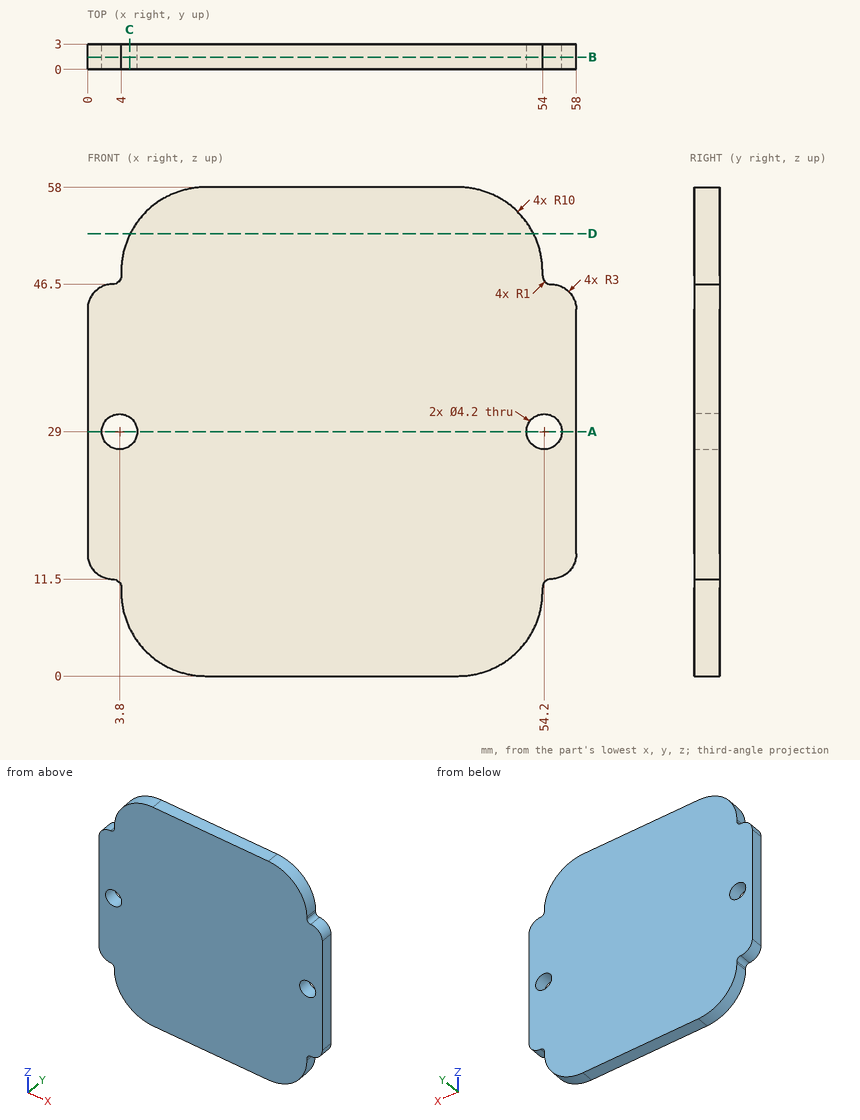
For this review, use the dimensioned drawing (mm, ordinates from the lowest corner) and the shaded views. Coordinates: 2 decimals unless noted, no trailing zeros. Loops run counter-clockwise (first coordinate to the right, second up) from the corner with the lowest first, then second, coordinate; pieces in that order, holes last. Notation, with made-up numbers: (-19.75, 57) - (-8.75, 57) arc R32 ccw to (-8.75, 88) - close; hole circle Ø6 at (26, -0.5). An arc over 180 degrees is marked (long way). Use one line per item in the form item = value. Start each with the question number.
1) Take a section at C-C (x = 5). State the section outline as (y, z) points, plus the area to 3 significant figures.
2) Take a section at B-B (y = 1.45). State how many separate pieces and enclosed holes the cut face has, plus the area to 3 significant figures.
3) To check wall thickness, follow probe 1 along X at (y, z) = (1.4, 29); probe 2 along X at (y, z) = (0.8, 27.5); probe 3 along Z at (x, y) = (55.5, 2.8). State the ranges of each line that lie inside material, in increasing order. Write a range as from..to.
4) Take a section at A-A (z = 29). State the section outline as (x, y) points.
5) Take a section at D-D (z = 52.5). State the section outline as (x, y) points.
6) For pin 1 (1.5 mm diameter, centred on x = 8.5, y = 1, fed in from +Z); pin 2 (0.6 mm diameter, centred on y = 1.5, z = 47.5, fed in from -X), all flat-tipped, find the tip position at first contact; note any pin that passes through.
From the geometry:
q1.outline = (0, 5.64) - (3, 5.64) - (3, 27.28) - (0, 27.28) - close; (0, 30.72) - (3, 30.72) - (3, 52.36) - (0, 52.36) - close
q1.area = 130 mm2
q2.separate_pieces = 1
q2.enclosed_holes = 2
q2.area = 3,060 mm2
q3.probe_1 = 0..1.7, 5.9..52.1, 56.3..58
q3.probe_2 = 0..2.33, 5.27..52.73, 55.67..58
q3.probe_3 = 11.54..27.35, 30.65..46.46
q4.outline = (0, 0) - (1.7, 0) - (1.7, 3) - (0, 3) - close; (5.9, 0) - (52.1, 0) - (52.1, 3) - (5.9, 3) - close; (56.3, 0) - (58, 0) - (58, 3) - (56.3, 3) - close
q5.outline = (5.07, 0) - (52.93, 0) - (52.93, 3) - (5.07, 3) - close
q6.pin_1 = 56.8
q6.pin_2 = 3.95
